For this review, take the finished solid that the model builds, in its own axes (mm). Face numbers are marked on the shaded views. A direction names the side the tool comes from. Round coordinates to 2 decimals unless told otherwise and drop trailing zeros. Order: outer loops, then holes, each group sorted by start corner. A loop starts at its lowest first (then second) coordinate and runs counter-clockwise, first axis right, second up. Notation, with made-up numbers: (-6, 22) - (48, 22) arc R21 cw to (48, 57) - close; hole circle Ø10 at (78, -16). An arc over 180 degrees is marked (long way). One line per item, written item: value.
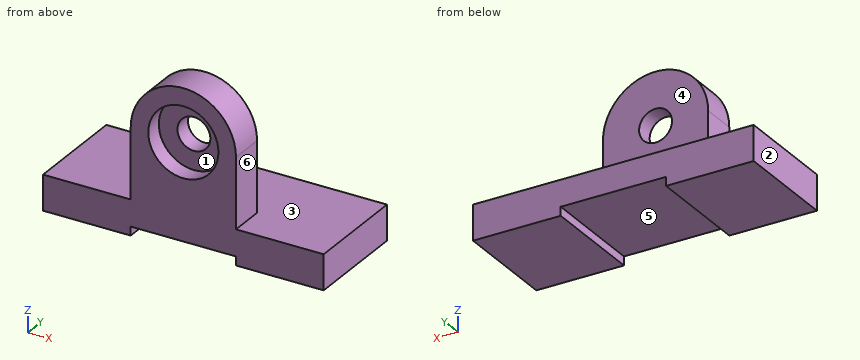
```python
from build123d import *

# Parameters (mm, degrees)
F0_W           = 101.6
F0_H           = 38.1
F1_DEPTH       = 12.7
F3_DEPTH       = 12.7
F4_D           = 11.90625
F4_CBORE_D     = 25.4
F4_CBORE_DEPTH = 6.35
F5_W           = 38.1
F5_H           = 3.175
F6_DEPTH       = 38.101


# Not quite as in the source:
# - a length typed as a fraction of an inch, garbled in the dataset ("3 / 203.2 mm" for 3/8 in), is restored


with BuildPart() as f1:
    # F0 (on Top) → F1 (new body)
    with BuildSketch(Plane.XY):
        with Locations((50.8, 19.05)):
            Rectangle(F0_W, F0_H)
    extrude(amount=F1_DEPTH)

    # F2 (on face) → F3 (join)
    with BuildSketch(Plane.XZ):
        with BuildLine():
            Line((31.75, 38.1), (31.75, 0))
            Line((31.75, 0), (69.85, 0))
            Line((69.85, 0), (69.85, 38.1))
            ThreePointArc((69.85, 38.1), (50.8, 57.15), (31.75, 38.1))
        make_face()
    extrude(amount=-F3_DEPTH)

    # F4 (through all)
    with Locations(Plane.XZ):
        with Locations((50.8, 38.1)):
            CounterBoreHole(F4_D / 2, F4_CBORE_D / 2, F4_CBORE_DEPTH)

    # F5 (on face) → F6 (cut, through all)
    with BuildSketch(Plane(origin=(0, 38.1, 0), x_dir=(-1, 0, 0), z_dir=(0, 1, 0))):
        with Locations((-50.8, 1.5875)):
            Rectangle(F5_W, F5_H)
    extrude(amount=-F6_DEPTH, mode=Mode.SUBTRACT)


solid = f1.part
```
Item 1: Take a section at D-D (x = 23). Write out the cut boundary in (y, z).
Returned:
outline: (0, 0) - (38.1, 0) - (38.1, 12.7) - (0, 12.7) - close
Item 2: Wall thickness on line 1 (Z direction, x = 50.8, y = 4) (3 decimals); line 2 (Z direction, x = 50.8, y = 9.5) (3 decimals); line 3 (Z direction, x = 45.5, y = 17) (3 decimals): over which ranges is each line inside the solid? List them lowest first.
Returned:
line 1: 3.175 to 25.4, 50.8 to 57.15
line 2: 3.175 to 32.147, 44.053 to 57.15
line 3: 3.175 to 12.7
Item 3: The part is to be moulded in two halves that separate along X. For the marked faces 1, 2 and 3, say which applies: +X half, -X half, draft (parallel to the pull), parting line (faces both ways), or undercut.
Returned:
face 1: undercut
face 2: -X half
face 3: draft
Item 4: Take a section at C-C (y = 34). Write out the cut boundary in (x, z) (3 decimals).
Returned:
outline: (0, 0) - (31.75, 0) - (31.75, 3.175) - (69.85, 3.175) - (69.85, 0) - (101.6, 0) - (101.6, 12.7) - (0, 12.7) - close
Item 5: Take a section at A-A (x = 50.8). Write out the cut boundary in (y, z) (3 decimals), plus the area to 3 significant figures.
Returned:
outline: (0, 3.175) - (38.1, 3.175) - (38.1, 12.7) - (12.7, 12.7) - (12.7, 32.147) - (6.35, 32.147) - (6.35, 25.4) - (0, 25.4) - close; (0, 50.8) - (6.35, 50.8) - (6.35, 44.053) - (12.7, 44.053) - (12.7, 57.15) - (0, 57.15) - close
area: 691 mm^2
Item 6: Machinability: for the marked faces 4, 5 and 6, which of the approach directions +Z, -Z, +X, -X, +Y, -Y give a long, thin tool a straight path to every point of the face, cutting with its end or side? Answer none if there is none.
Returned:
face 4: +Z, +X, -X, +Y
face 5: -Z, +Y, -Y
face 6: +Z, +X, +Y, -Y
Item 7: Take a section at B-B (z = 28). Write out the cut boundary in (x, y), plus the area to 3 significant figures.
Returned:
outline: (31.75, 0) - (43.1, 0) - (43.1, 6.35) - (58.5, 6.35) - (58.5, 0) - (69.85, 0) - (69.85, 12.7) - (31.75, 12.7) - close
area: 386 mm^2
Item 8: For P1, Ø19, axis at x = 53, z = 30.5, coming from the +Y side; P2, Ø2, axis at x = 48.5, y = 32, coming from the -Z side (3 decimals); P3, Ø19, axis at x = 45, y = 17, coming from the +Z side, all flat-tipped, find the tip position at first contact; note any pin that passes through.
Returned:
P1: y = 12.7
P2: z = 3.175
P3: z = 57.15
